Verification items for the finished model (mm, model axes). Face numbers are marked on the shaded views. Give positions to 0.01 mm unless a question says otherwise; leave off trailing zeros. Loops run counter-clockwise (first coordinate to the right, second up) from the corner with the lowest first, then second, coordinate; pieces in that order, holes last. Notation, with made-up numbers: (36.25, -30.75) - (71.25, -30.75) arc R25 cw to (71.25, 2.25) - close; hole circle Ø5 at (59.5, 1.5). An arc over 180 degrees is marked (long way). Put each result on its own line as item: value. Start each with the question number.
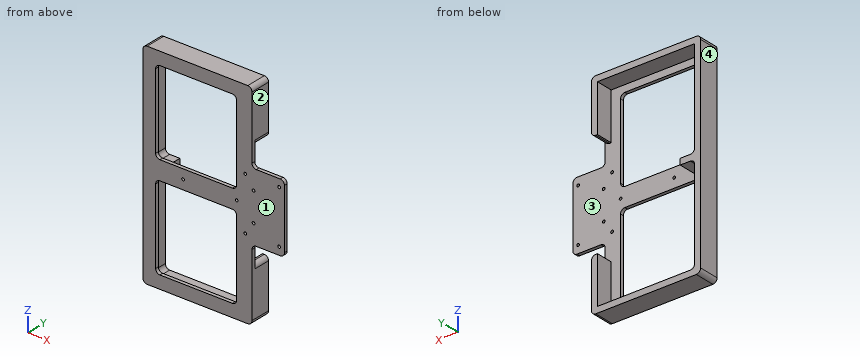
```python
from build123d import *

# Parameters (mm, degrees)
SKETCH1_R           = 1.6
BOSS_EXTRUDE1_DEPTH = 2
BOSS_EXTRUDE2_DEPTH = 20
FILLET1_R           = 5


with BuildPart() as part:
    # Sketch1 → Boss-Extrude1 (new body, symmetric)
    with BuildSketch(Plane(origin=(0, 0, 0), x_dir=(1, 0, 0), z_dir=(0, 1, 0))):
        Polygon((18, 40), (56, 40), (56, -40), (18, -40), (18, -124), (-110, -124), (-110, -22.904637916), (-110, 22.904637916), (-110, 124), (18, 124), align=None)
        Circle(SKETCH1_R, mode=Mode.SUBTRACT)
        with Locations((-62.8, 0)):
            Circle(SKETCH1_R, mode=Mode.SUBTRACT)
        with Locations((10, 31)):
            Circle(SKETCH1_R, mode=Mode.SUBTRACT)
        with Locations((49.8, 31)):
            Circle(SKETCH1_R, mode=Mode.SUBTRACT)
        with Locations((49.8, -31)):
            Circle(SKETCH1_R, mode=Mode.SUBTRACT)
        with Locations((10, -31)):
            Circle(SKETCH1_R, mode=Mode.SUBTRACT)
        with Locations((19.8, 17)):
            Circle(SKETCH1_R, mode=Mode.SUBTRACT)
        with Locations((19.8, -17)):
            Circle(SKETCH1_R, mode=Mode.SUBTRACT)
        Polygon((0, 11), (-95, 11), (-95, 109), (0, 109), (0, 40), align=None, mode=Mode.SUBTRACT)
        Polygon((0, -11), (0, -40), (0, -109), (-95, -109), (-95, -11), align=None, mode=Mode.SUBTRACT)
    extrude(amount=BOSS_EXTRUDE1_DEPTH, both=True)

    # Sketch2 → Boss-Extrude2 (add)
    with BuildSketch(Plane(origin=(0, 2, 0), x_dir=(1, 0, 0), z_dir=(0, 1, 0))):
        Polygon((18, 124), (-110, 124), (-110, -124), (18, -124), (18, -117), (18, -62), (11, -62), (11, -117), (-103, -117), (-103, -3.5), (-86, -3.5), (-86, 3.5), (-103, 3.5), (-103, 117), (11, 117), (11, 62), (18, 62), (18, 117), align=None)
    extrude(amount=BOSS_EXTRUDE2_DEPTH)

    # Fillet1
    fillet1_edges = [part.edges().sort_by_distance(p)[0] for p in [
        (18, 12, 62),
        (-103, 12, 3.5),
        (-103, 12, -3.5),
        (-103, 12, -117),
        (18, 12, -62),
        (18, 0, 40),
        (18, 10, 124),
        (-110, 10, 124),
        (-110, 10, -124),
        (18, 10, -124),
        (18, 0, -40),
        (56, 0, -40),
        (56, 0, 40),
        (0, 0, -11),
        (0, 0, -109),
        (-95, 0, -109),
        (-95, 0, -11),
        (0, 0, 11),
        (-95, 0, 11),
        (-95, 0, 109),
        (0, 0, 109),
    ]]
    fillet(fillet1_edges, radius=FILLET1_R)


solid = part.part
```
1) Draft check along X on the marked faces 1, 2, 3 and 4. Enter one of: pulls with the +X half, pulls with the -X half, needs draft (parallel to the pull), parting line crosses it, or undercut.
2) Scan lines: line 1 along X through (y, z) = (-0.25, 0); line 2 along Z through (x, y) = (-62.8, 0.7); line 3 along X through (y, z) = (1.15, -31). Record each from-to range of solid material in increasing order. Write a range as from..to.
3) Section check C-C, the plane y = 18.75. Enter the section's corners in (x, z).
4) Depth check by flat-ended pin: P1, Ø3, axis at y = 4.5, z = 36.5, coming from the +X side; P2, Ø1.5, axis at x = -83.5, z = 7.5, coming from the +Y side; P3, Ø2, axis at y = 10.5, z = -1.5, coming from the +X side. Enter the tip coordinate at first touch or a pass-through.
5) Section check B-B, the plane z = -92. Enter the section's corners in (x, y), plus the area to 3 significant figures.
6) Section check A-A, the plane x = -39. Enter the section's corners in (y, z), plus the area to 3 significant figures.
7) Section check D-D, the plane z = -37.5. Enter the section's corners in (x, y).
Results are:
1. face 1: needs draft
1. face 2: pulls with the +X half
1. face 3: undercut
1. face 4: pulls with the -X half
2. line 1: x = -110..-64.4, -61.2..-1.6, 1.6..56
2. line 2: z = -124..-109, -11..-1.6, 1.6..11, 109..124
2. line 3: x = -110..-95, 0..8.4, 11.6..48.2, 51.4..56
3. outline: (-110, -119) arc R5 ccw to (-105, -124) - (13, -124) arc R5 ccw to (18, -119) - (18, -67) arc R5 ccw to (13, -62) - (11, -62) - (11, -117) - (-98, -117) arc R5 cw to (-103, -112) - (-103, -8.5) arc R5 cw to (-98, -3.5) - (-86, -3.5) - (-86, 3.5) - (-98, 3.5) arc R5 cw to (-103, 8.5) - (-103, 117) - (11, 117) - (11, 62) - (13, 62) arc R5 ccw to (18, 67) - (18, 119) arc R5 ccw to (13, 124) - (-105, 124) arc R5 ccw to (-110, 119) - close
4. P1: stops at x = -103
4. P2: stops at y = 2
4. P3: stops at x = -86
5. outline: (-110, -2) - (-95, -2) - (-95, 2) - (-103, 2) - (-103, 22) - (-110, 22) - close; (0, -2) - (18, -2) - (18, 22) - (11, 22) - (11, 2) - (0, 2) - close
5. area: 412 mm2
6. outline: (-2, -124) - (22, -124) - (22, -117) - (2, -117) - (2, -109) - (-2, -109) - close; (-2, -11) - (2, -11) - (2, 11) - (-2, 11) - close; (-2, 109) - (2, 109) - (2, 117) - (22, 117) - (22, 124) - (-2, 124) - close
6. area: 488 mm2
7. outline: (-110, -2) - (-95, -2) - (-95, 2) - (-103, 2) - (-103, 22) - (-110, 22) - close; (0, -2) - (55.33, -2) - (55.33, 2) - (0, 2) - close
